from build123d import *

# Parameters (mm, degrees)
SKETCH1_W            = 58
SKETCH1_H            = 80
BOSS_EXTRUDE1_DEPTH  = 4
CUT_EXTRUDE1_DEPTH   = 25
SKETCH5_W            = 13
SKETCH5_H            = 16
BOSS_EXTRUDE3_DEPTH  = 80
SKETCH6_R            = 2.53
CUT_EXTRUDE2_DEPTH   = 59
SKETCH7_R            = 4.53
SKETCH7_R_2          = 2.53
BOSS_EXTRUDE4_DEPTH  = 1
SKETCH8_R            = 1.8
CUT_EXTRUDE3_DEPTH   = 21
SKETCH9_W            = 8
SKETCH9_H            = 80
CUT_EXTRUDE4_DEPTH   = 7.6
SKETCH13_W           = 6
SKETCH13_H           = 4.261
BOSS_EXTRUDE6_DEPTH  = 11.35
SKETCH14_W           = 6
SKETCH14_H           = 16
BOSS_EXTRUDE7_DEPTH  = 8
SKETCH15_W           = 40
SKETCH15_H           = 4.261
BOSS_EXTRUDE8_DEPTH  = 19.35
FILLET1_R            = 10
FILLET2_R            = 3
FILLET3_R            = 3
SKETCH17_W           = 17
SKETCH17_H           = 24
CUT_EXTRUDE6_DEPTH   = 5
FILLET4_R            = 14
FILLET5_R            = 4
FILLET6_R            = 2
FILLET7_R            = 0.5
BOSS_EXTRUDE10_DEPTH = 2
SKETCH19_W           = 58
SKETCH19_H           = 5.571501033
SKETCH19_H_2         = 14.101029475
CUT_EXTRUDE7_DEPTH   = 21
SKETCH20_W           = 96.7
SKETCH20_H           = 30
CUT_EXTRUDE8_DEPTH   = 21.0000001
CUT_EXTRUDE9_DEPTH   = 16


with BuildPart() as part:
    # Sketch1 → Boss-Extrude1 (new body)
    with BuildSketch(Plane(origin=(0, 0, 0), x_dir=(1, 0, 0), z_dir=(0, 1, 0))):
        Rectangle(SKETCH1_W, SKETCH1_H)
    extrude(amount=BOSS_EXTRUDE1_DEPTH)

    # Sketch2 → Cut-Extrude1 (cut)
    with BuildSketch(Plane.ZY.offset(29)):
        Polygon((1.834230855, 4), (-1.834230855, 4), (-3, 1.5), (3, 1.5), align=None)
        Polygon((8.165769145, 4), (11.834230855, 4), (13, 1.5), (7, 1.5), align=None)
        Polygon((-7, 1.5), (-8.165769145, 4), (-11.834230855, 4), (-13, 1.5), align=None)
    extrude(amount=-CUT_EXTRUDE1_DEPTH, mode=Mode.SUBTRACT)

    # Sketch5 → Boss-Extrude3 (add)
    with BuildSketch(Plane.XY.offset(40)):
        with Locations((22.5, 12)):
            Rectangle(SKETCH5_W, SKETCH5_H)
    extrude(amount=-BOSS_EXTRUDE3_DEPTH)

    # Sketch6 → Cut-Extrude2 (cut, through all)
    with BuildSketch(Plane(origin=(29, 0, 0), x_dir=(0, 0, -1), z_dir=(1, 0, 0))):
        with Locations((0, 12)):
            Circle(SKETCH6_R)
    extrude(amount=-CUT_EXTRUDE2_DEPTH, mode=Mode.SUBTRACT)

    # Sketch7 → Boss-Extrude4 (add)
    with BuildSketch(Plane(origin=(29, 0, 0), x_dir=(0, 0, -1), z_dir=(1, 0, 0))):
        with Locations((0, 12)):
            Circle(SKETCH7_R)
        with Locations((0, 12)):
            Circle(SKETCH7_R_2, mode=Mode.SUBTRACT)
    extrude(amount=BOSS_EXTRUDE4_DEPTH)

    # Sketch8 → Cut-Extrude3 (cut, through all)
    with BuildSketch(Plane(origin=(0, 20, 0), x_dir=(1, 0, 0), z_dir=(0, 1, 0))):
        with Locations((22.5, 6.7)):
            Circle(SKETCH8_R)
        with Locations((22.5, -6.7)):
            Circle(SKETCH8_R)
    extrude(amount=-CUT_EXTRUDE3_DEPTH, mode=Mode.SUBTRACT)

    # Sketch9 → Cut-Extrude4 (cut)
    with BuildSketch(Plane.XZ):
        with Locations((22.5, 0)):
            Rectangle(SKETCH9_W, SKETCH9_H)
    extrude(amount=-CUT_EXTRUDE4_DEPTH, mode=Mode.SUBTRACT)

    # Sketch13 → Boss-Extrude6 (add)
    with BuildSketch(Plane(origin=(29, 0, 0), x_dir=(0, 0, -1), z_dir=(1, 0, 0))):
        with Locations((0, 2.1305)):
            Rectangle(SKETCH13_W, SKETCH13_H)
    extrude(amount=BOSS_EXTRUDE6_DEPTH)

    # Sketch14 → Boss-Extrude7 (add)
    with BuildSketch(Plane(origin=(40.35, 0, 0), x_dir=(0, 0, -1), z_dir=(1, 0, 0))):
        with Locations((0, 8)):
            Rectangle(SKETCH14_W, SKETCH14_H)
    extrude(amount=BOSS_EXTRUDE7_DEPTH)

    # Sketch15 → Boss-Extrude8 (add)
    with BuildSketch(Plane(origin=(29, 0, 0), x_dir=(0, 0, -1), z_dir=(1, 0, 0))):
        with Locations((0, 2.1305)):
            Rectangle(SKETCH15_W, SKETCH15_H)
    extrude(amount=BOSS_EXTRUDE8_DEPTH)

    # Fillet1
    fillet1_edges = [part.edges().sort_by_distance(p)[0] for p in [
        (44.35, 4.261, 3),
        (44.35, 4.261, -3),
    ]]
    fillet(fillet1_edges, radius=FILLET1_R)

    # Fillet2
    fillet2_edges = [part.edges().sort_by_distance(p)[0] for p in [
        (29, 4.261, 0),
    ]]
    fillet(fillet2_edges, radius=FILLET2_R)

    # Fillet3
    fillet3_edges = [part.edges().sort_by_distance(p)[0] for p in [
        (29, 2.1305, -20),
        (29, 2.1305, 20),
    ]]
    fillet(fillet3_edges, radius=FILLET3_R)

    # Sketch17 → Cut-Extrude6 (cut, through all)
    with BuildSketch(Plane(origin=(0, 4, 0), x_dir=(1, 0, 0), z_dir=(0, 1, 0))):
        with Locations((7.5, -24)):
            Rectangle(SKETCH17_W, SKETCH17_H)
        with Locations((7.5, 24)):
            Rectangle(SKETCH17_W, SKETCH17_H)
    extrude(amount=-CUT_EXTRUDE6_DEPTH, mode=Mode.SUBTRACT)

    # Fillet4
    fillet4_edges = [part.edges().sort_by_distance(p)[0] for p in [
        (16, 4, 38),
        (16, 4, -38),
    ]]
    fillet(fillet4_edges, radius=FILLET4_R)

    # Fillet5
    fillet5_edges = [part.edges().sort_by_distance(p)[0] for p in [
        (16, 4, 0),
    ]]
    fillet(fillet5_edges, radius=FILLET5_R)

    # Fillet6
    fillet6_edges = [part.edges().sort_by_distance(p)[0] for p in [
        (16, 6, 12),
        (16, 11, 36),
        (16, 11, -36),
        (16, 6, -12),
    ]]
    fillet(fillet6_edges, radius=FILLET6_R)

    # Fillet7
    fillet7_edges = [part.edges().sort_by_distance(p)[0] for p in [
        (-16.5, 4, -11.834230855),
        (-16.5, 4, -8.165769145),
        (-16.5, 4, 8.165769145),
        (-16.5, 4, 11.834230855),
        (-16.5, 4, 1.834230855),
        (-16.5, 4, -1.834230855),
    ]]
    fillet(fillet7_edges, radius=FILLET7_R)

    # Sketch18 → Boss-Extrude10 (add)
    with BuildSketch(Plane.XZ.offset(-7.6)):
        Polygon((20.016762412, 40.30109367), (24.983237588, 40.30109367), (27.466475177, 36), (24.983237588, 31.69890633), (20.016762412, 31.69890633), (17.533524823, 36), align=None)
        Polygon((20.882787815, 38.80109367), (24.117212185, 38.80109367), (25.734424369, 36), (24.117212185, 33.19890633), (20.882787815, 33.19890633), (19.265575631, 36), align=None, mode=Mode.SUBTRACT)
        Polygon((20.016762412, 11.00109367), (24.983237588, 11.00109367), (27.466475177, 6.7), (24.983237588, 2.39890633), (20.016762412, 2.39890633), (17.533524823, 6.7), align=None)
        Polygon((20.882787815, 9.50109367), (24.117212185, 9.50109367), (25.734424369, 6.7), (24.117212185, 3.89890633), (20.882787815, 3.89890633), (19.265575631, 6.7), align=None, mode=Mode.SUBTRACT)
        Polygon((20.016762412, -2.39890633), (24.983237588, -2.39890633), (27.466475177, -6.7), (24.983237588, -11.00109367), (20.016762412, -11.00109367), (17.533524823, -6.7), align=None)
        Polygon((20.882787815, -3.89890633), (24.117212185, -3.89890633), (25.734424369, -6.7), (24.117212185, -9.50109367), (20.882787815, -9.50109367), (19.265575631, -6.7), align=None, mode=Mode.SUBTRACT)
        Polygon((20.016762412, -31.69890633), (24.983237588, -31.69890633), (27.466475177, -36), (24.983237588, -40.30109367), (20.016762412, -40.30109367), (17.533524823, -36), align=None)
        Polygon((20.882787815, -33.19890633), (24.117212185, -33.19890633), (25.734424369, -36), (24.117212185, -38.80109367), (20.882787815, -38.80109367), (19.265575631, -36), align=None, mode=Mode.SUBTRACT)
    extrude(amount=BOSS_EXTRUDE10_DEPTH)

    # Sketch19 → Cut-Extrude7 (cut, through all)
    with BuildSketch(Plane.XZ):
        with Locations((0, -42.785750517)):
            Rectangle(SKETCH19_W, SKETCH19_H)
        with Locations((0, 47.050514738)):
            Rectangle(SKETCH19_W, SKETCH19_H_2)
    extrude(amount=-CUT_EXTRUDE7_DEPTH, mode=Mode.SUBTRACT)

    # Sketch20 → Cut-Extrude8 (cut, through all)
    with BuildSketch(Plane(origin=(0, 20, 0), x_dir=(1, 0, 0), z_dir=(0, 1, 0))):
        with Locations((0, 25)):
            Rectangle(SKETCH20_W, SKETCH20_H)
        with Locations((0, -25)):
            Rectangle(SKETCH20_W, SKETCH20_H)
    extrude(amount=-CUT_EXTRUDE8_DEPTH, mode=Mode.SUBTRACT)

    # Sketch22 → Cut-Extrude9 (cut)
    with BuildSketch(Plane.ZY.offset(4)):
        with BuildLine():
            Line((-10, 4), (-10, 1.5))
            Line((-10, 1.5), (-7, 1.5))
            Line((-7, 1.5), (-7.83408025, 3.288690869))
            ThreePointArc((-7.83408025, 3.288690869), (-7.80262208, 3.768649804), (-7.380926357, 4))
            Line((-7.380926357, 4), (-10, 4))
        make_face()
        with BuildLine():
            Line((3, 1.5), (2.16591975, 3.288690869))
            ThreePointArc((2.16591975, 3.288690869), (2.19737792, 3.768649804), (2.619073643, 4))
            Line((2.619073643, 4), (-2.619073643, 4))
            ThreePointArc((-2.619073643, 4), (-2.19737792, 3.768649804), (-2.16591975, 3.288690869))
            Line((-2.16591975, 3.288690869), (-3, 1.5))
            Line((-3, 1.5), (3, 1.5))
        make_face()
        with BuildLine():
            Line((7, 1.5), (10, 1.5))
            Line((10, 1.5), (10, 4))
            Line((10, 4), (7.380926357, 4))
            ThreePointArc((7.380926357, 4), (7.80262208, 3.768649804), (7.83408025, 3.288690869))
            Line((7.83408025, 3.288690869), (7, 1.5))
        make_face()
    extrude(amount=-CUT_EXTRUDE9_DEPTH, mode=Mode.SUBTRACT)


solid = part.part
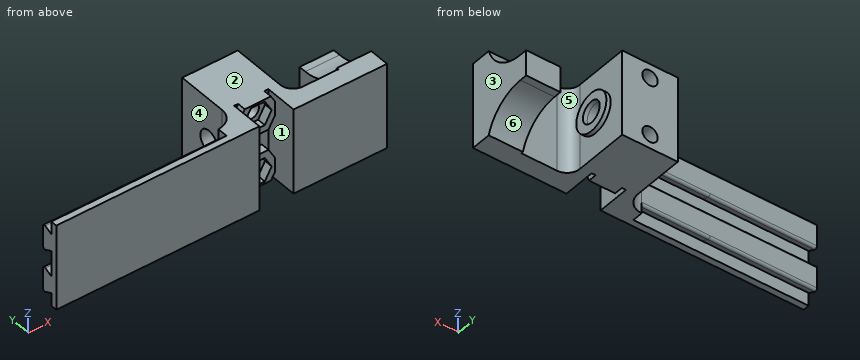
Check sheet for the modelled part. Datum: model origin and axes. Units: mm. Face numbers are marked on the shaded views. A direction names the side the tool comes from. Coordinates: 2 decimals unless noted, no trailing zeros. Loops run counter-clockwise (first coordinate to the right, second up) from the corner with the lowest first, then second, coordinate; pieces in that order, holes last. Notation, with made-up numbers: (79, 75.25) -> (87, 75.25) arc R18 cw to (87, 90.25) -> close; hole circle Ø3 at (87.5, 24.5). An arc over 180 degrees is marked (long way). Write item = value, one per line. Start each with the question number.
1. Depth check by flat-ended pin: P1, Ø6, axis at x = 22.5, z = -6, coming from the -Y side; P2, Ø1, axis at x = -10.5, z = 2.5, coming from the +Y side; P3, Ø1.5, axis at x = -4.5, z = -3.5, coming from the -Y side; P4, Ø3, axis at x = -3.5, z = 0.5, coming from the +Y side. Enter the tip coordinate at first touch or a pass-through.
2. Section check A-A on x = 22.5. Record the cut outline in (y, z), then the cut area to 3 significant figures.
3. Section check B-B on z = 0. Record the cut outline in (x, y), then the cut area to 3 significant figures.
4. Tool access check on the marked faces 4, 5 and 6. Record the directions out of +Z, -Z, +X, -X, +Y, -Y that give a thin tool (end or side, any length) a straight path to the whole face; none if there is none.
5. Section check C-C on y = 12. Record the cut outline in (x, z).
6. Section check D-D on x = 5. Record the cut outline in (y, z), then the cut area to 3 significant figures.
7. Material ranges on line 1 (Z direction, x = 22.5, y = 17); line 2 (X direction, y = 1.5, z = -4.25); line 3 (Y direction, x = 26.25, z = 0), recorded low to high.
8. Draft check along X on the marked faces 1, 2 and 3. Enter one of: released by +X, released by -X, zero draft, split by the parting line, or undercut.
Responses:
q1.P1 = 5.6
q1.P2 = 4
q1.P3 = 0
q1.P4 = 1.5
q2.outline = (5.6, -10) -> (20, -10) -> (20, -8.5) -> (7.6, -8.5) -> (7.6, -9.5) -> (5.6, -9.5) -> close; (5.6, -3.9) -> (7.6, -3.9) -> (7.6, -4.9) -> (20, -4.9) -> (20, 4.9) -> (7.6, 4.9) -> (7.6, 3.9) -> (5.6, 3.9) -> (5.6, 2.4) -> (7.6, 2.4) -> (7.6, -2.4) -> (5.6, -2.4) -> close; (5.6, 9.5) -> (7.6, 9.5) -> (7.6, 8.5) -> (20, 8.5) -> (20, 10) -> (5.6, 10) -> close; hole circle Ø5.06 at (12, 0)
q2.area = 147 mm2
q3.outline = (-29, 0) -> (18.5, 0) -> (18.5, 7.6) -> (26.5, 7.6) -> (26.5, 0) -> (48.35, 0) -> (48.35, 16) -> (40.35, 16) -> (40.35, 4.26) -> (32, 4.26) arc R3 cw to (29, 7.26) -> (29, 7.47) -> (30, 7.47) -> (30, 9.47) -> (16, 9.47) -> (16, 8) arc R4 cw to (12, 4) -> (12, 1.5) -> (-29, 1.5) -> close; (16, 14.53) -> (30, 14.53) -> (30, 16.53) -> (29, 16.53) -> (29, 20) -> (16, 20) -> close
q3.area = 397 mm2
q4.face_4 = +Z, -Z, -X, +Y
q4.face_5 = +Z, -Z
q4.face_6 = -Z, +X, +Y
q5.outline = (16, -10) -> (29, -10) -> (29, -4.53) -> (30, -4.53) -> (30, -2.53) -> (16, -2.53) -> close; (16, 2.53) -> (30, 2.53) -> (30, 4.53) -> (29, 4.53) -> (29, 10) -> (16, 10) -> close; (40.35, -3.26) -> (48.35, -3.26) -> (48.35, 3.26) -> (40.35, 3.26) -> close; hole circle Ø3.6 at (22.5, -6.7); hole circle Ø3.6 at (22.5, 6.7)
q6.outline = (0, -10) -> (1.5, -10) -> (1.5, -7) -> (3.29, -7.83) arc R0.5 ccw to (4, -7.38) -> (4, -2.62) arc R0.5 ccw to (3.29, -2.17) -> (1.5, -3) -> (1.5, 3) -> (3.29, 2.17) arc R0.5 ccw to (4, 2.62) -> (4, 7.38) arc R0.5 ccw to (3.29, 7.83) -> (1.5, 7) -> (1.5, 10) -> (0, 10) -> close
q6.area = 55.3 mm2
q7.line_1 = -10 to -8.5, -4.9 to 4.9, 8.5 to 10
q7.line_2 = -29 to 18.5, 26.5 to 48.35
q7.line_3 = 7.6 to 9.47, 14.53 to 20
q8.face_1 = undercut
q8.face_2 = zero draft
q8.face_3 = released by +X
